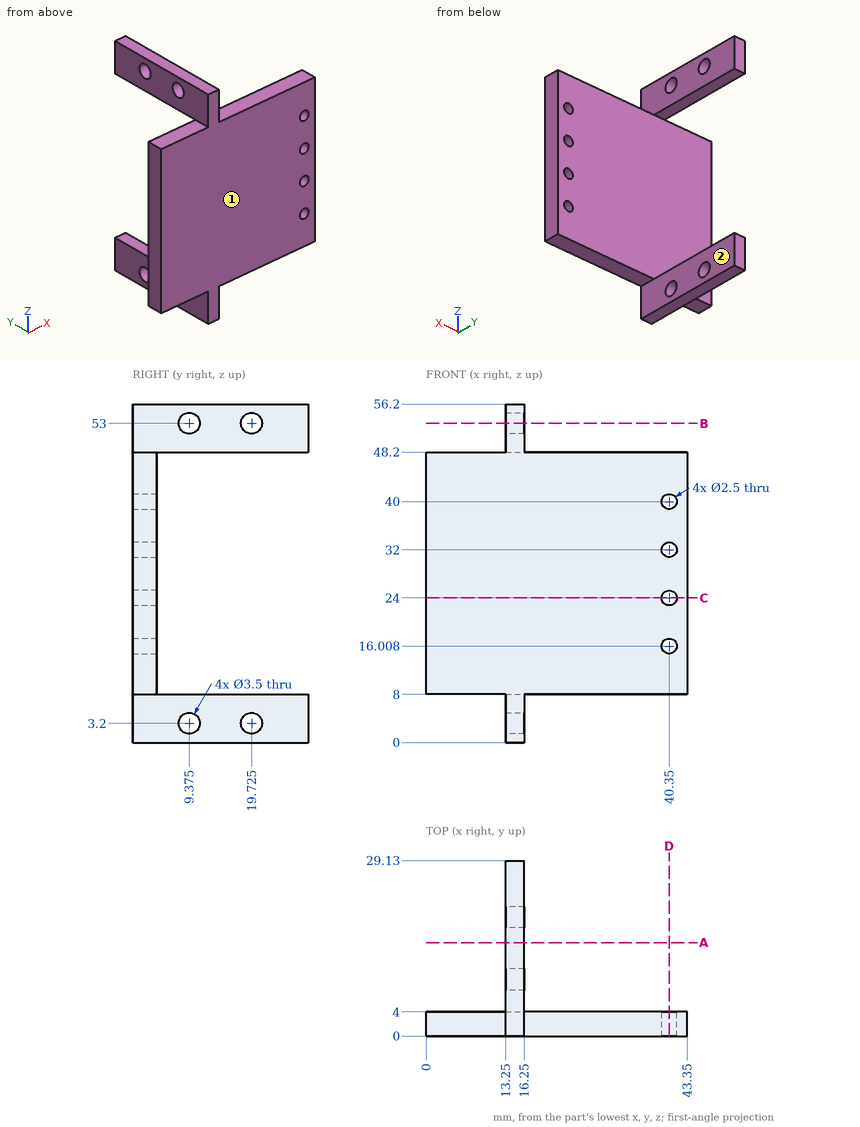
Design review of the part shown in the three views and the two pictorial views. Dimensions are in mm from the part's minimum x, y and z. A direction names the side the tool comes from. Round coordinates to 2 decimals unless told otherwise and drop trailing zeros. Order: outer loops, then holes, each group sorted by start corner. A loop starts at its lowest first (then second) coordinate and runs counter-clockwise, first axis right, second up. Notation, with made-up numbers: (58.25, 15.5) - (93.25, 15.5) arc R23 cw to (93.25, 23.5) - close; hole circle Ø6 at (18.25, 30). An arc over 180 degrees is marked (long way). Answer in a Markdown table with one row per item.
(1) Take a section at C-C on z = 24. Write out the cut boundary in (x, y).
Result set:
| item | result |
|---|---|
| outline | (0, 0) - (39.1, 0) - (39.1, 4) - (0, 4) - close; (41.6, 0) - (43.35, 0) - (43.35, 4) - (41.6, 4) - close |
(2) Take a section at B-B on z = 53. Write out the cut boundary in (x, y) (3 decimals), plus the area to 3 significant figures.
Result set:
| item | result |
|---|---|
| outline | (13.25, 0) - (16.25, 0) - (16.25, 7.625) - (13.25, 7.625) - close; (13.25, 11.125) - (16.25, 11.125) - (16.25, 17.975) - (13.25, 17.975) - close; (13.25, 21.475) - (16.25, 21.475) - (16.25, 29.13) - (13.25, 29.13) - close |
| area | 66.4 mm2 |
(3) Take a section at D-D on x = 40.35. Write out the cut boundary in (y, z).
Result set:
| item | result |
|---|---|
| outline | (0, 8) - (4, 8) - (4, 14.76) - (0, 14.76) - close; (0, 17.26) - (4, 17.26) - (4, 22.75) - (0, 22.75) - close; (0, 25.25) - (4, 25.25) - (4, 30.75) - (0, 30.75) - close; (0, 33.25) - (4, 33.25) - (4, 38.75) - (0, 38.75) - close; (0, 41.25) - (4, 41.25) - (4, 48.2) - (0, 48.2) - close |
(4) Clearance check with flat-ended pins moving along their axes: P1, Ø3, axis at y = 19.725, z = 3.2, coming from the +X side; P2, Ø4, axis at y = 18, z = 51.5, coming from the +X side; P3, Ø4.5, axis at y = 9.375, z = 3.2, coming from the -X side; P4, Ø3, axis at x = 40.35, z = 24, coming from the +Y side. State where each tip first meets the part, or that it passes through.
Result set:
| item | result |
|---|---|
| P1 | passes through |
| P2 | stops at x = 16.25 |
| P3 | stops at x = 13.25 |
| P4 | stops at y = 4 |
(5) Machinability: for the marked faces 1 and 2, which of the approach directions +Z, -Z, +X, -X, +Y, -Y give a long, thin tool a straight path to every point of the face, cutting with its end or side? Answer none if there is none.
Result set:
| item | result |
|---|---|
| face 1 | +Z, -Z, +X, -X, -Y |
| face 2 | -Z, +X, +Y, -Y |
(6) For line 1 (Y direction, x = 14.85, z = 53) (3 decimals); line 2 (Z direction, x = 40.35, y = 1.1); line 3 (X direction, y = 2.2, z = 32), list the stretches that pass through material, from the lowest coordinate up. Write a range as from..to.
Result set:
| item | result |
|---|---|
| line 1 | y = 0..7.625, 11.125..17.975, 21.475..29.13 |
| line 2 | z = 8..14.76, 17.26..22.75, 25.25..30.75, 33.25..38.75, 41.25..48.2 |
| line 3 | x = 0..39.1, 41.6..43.35 |
(7) Take a section at A-A on y = 15.5. Write out the cut boundary in (x, z).
Result set:
| item | result |
|---|---|
| outline | (13.25, 0) - (16.25, 0) - (16.25, 8) - (13.25, 8) - close; (13.25, 48.2) - (16.25, 48.2) - (16.25, 56.2) - (13.25, 56.2) - close |
